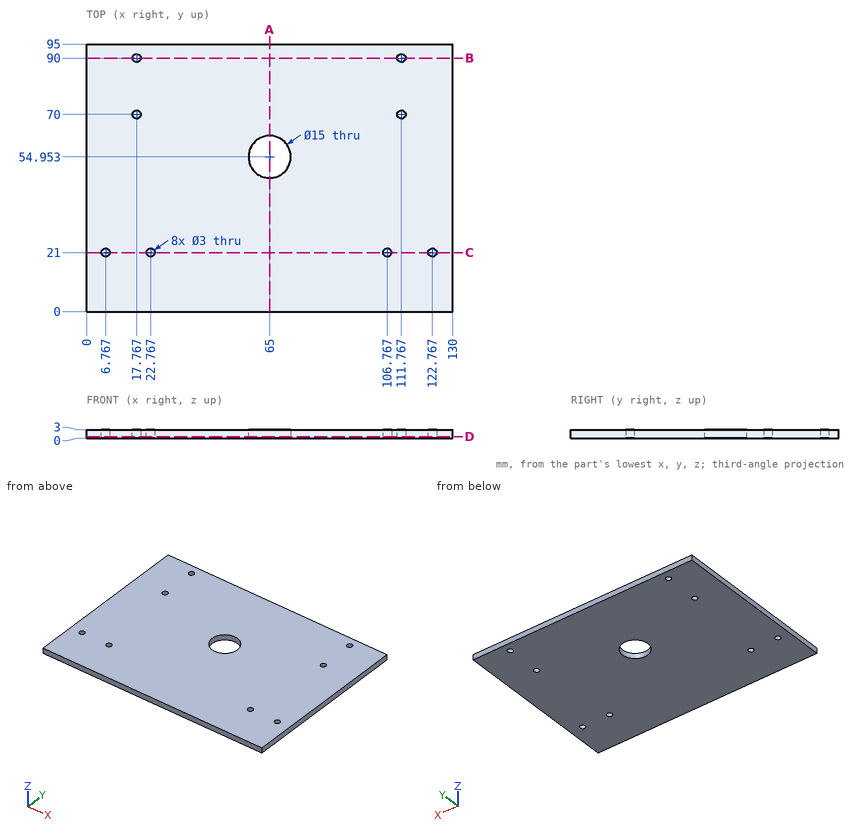
Study the drawing (mm; zero at the part's minimum x, y, z) and answer. Round coordinates to 2 decimals unless told otherwise and drop trailing zeros. Write each loop counter-clockwise with the first axis right and the second up, starting at its lowest first coordinate (ties: lowest second). Pieces come first, ordered by that corner, then holes. Notation, with made-up numbers: (-11.75, -15.75) - (1.25, -15.75) arc R19 cw to (1.25, 8.25) - close; hole circle Ø6 at (-17.75, -7). An arc over 180 degrees is marked (long way). Return JSON: item names as keys, results as strings. Group by question number.
Q1. The part is cut by section A-A on x = 65. Write down the section's boundary in (y, z), then the cut area to 3 significant figures.
Q2. The part is cut by section B-B on y = 90. Write down the section's boundary in (x, z), then the cut area to 3 significant figures.
Q3. The part is cut by section C-C on y = 21. Write down the section's boundary in (x, z).
Q4. Find the intervals of material crossed by L1, parallel to X at y = 70, z = 1.95; L2, parallel to X at y = 69.5, z = 1.8; L3, parallel to X at y = 61, z = 1.05 (1 decimal), in increasing order.
Q5. The part is cut by section D-D on z = 0.55. Count the separate pieces of the cut face and the enclosed holes in it, then the cut area to 3 significant figures.
Solved:
{
 "1": {"outline": "(0, 0) - (47.45, 0) - (47.45, 3) - (0, 3) - close; (62.45, 0) - (95, 0) - (95, 3) - (62.45, 3) - close", "area": "240 mm²"},
 "2": {"outline": "(0, 0) - (16.27, 0) - (16.27, 3) - (0, 3) - close; (19.27, 0) - (110.27, 0) - (110.27, 3) - (19.27, 3) - close; (113.27, 0) - (130, 0) - (130, 3) - (113.27, 3) - close", "area": "372 mm²"},
 "3": {"outline": "(0, 0) - (5.27, 0) - (5.27, 3) - (0, 3) - close; (8.27, 0) - (21.27, 0) - (21.27, 3) - (8.27, 3) - close; (24.27, 0) - (105.27, 0) - (105.27, 3) - (24.27, 3) - close; (108.27, 0) - (121.27, 0) - (121.27, 3) - (108.27, 3) - close; (124.27, 0) - (130, 0) - (130, 3) - (124.27, 3) - close"},
 "4": {"L1": "0 to 16.27, 19.27 to 110.27, 113.27 to 130", "L2": "0 to 16.35, 19.18 to 110.35, 113.18 to 130", "L3": "0 to 60.6, 69.4 to 130"},
 "5": {"separate pieces": "1", "enclosed holes": "9", "area": "12,100 mm²"}
}
